Design review of the part built by this model. Coordinates are the model's own, in mm. Face numbers are marked on the shaded views. A direction names the side the tool comes from. Coordinates: 2 decimals unless noted, no trailing zeros. Write each loop counter-clockwise with the first axis right and the second up, starting at its lowest first coordinate (ties: lowest second). Pieces come first, ordered by that corner, then holes. Notation, with made-up numbers: M 74.25,16 L 118.25,16 A20 cw 118.25,37 Z; hole C 71,-16 d4. An arc over 180 degrees is marked long. Write item = value, one per line.
```python
from build123d import *

# Parameters (mm, degrees)
SKETCH1_R           = 1.8749999999999902
SKETCH1_R_2         = 1.8749999999999822
BOSS_EXTRUDE1_DEPTH = 50


with BuildPart() as part:
    # Sketch1 → Boss-Extrude1 (new body)
    # profile 1 of 3: a face of its own
    with BuildSketch(Plane.XY):
        with BuildLine():
            ThreePointArc((-544.9073445733862, 245.05934298496234), (-541.6610147269474, 238.65452406819674), (-534.9592100975257, 236.0765059267749))
            Line((-534.9592100975257, 236.07650592677487), (-441.5899759130262, 236.07650592677487))
            Line((-441.5899759130262, 236.07650592677484), (-439.06259783112466, 236.07650592677484))
            ThreePointArc((-439.06259783112466, 236.07650592677484), (-397.37358262088145, 226.97219345264216), (-363.27556383489673, 201.31702614277702))
            add(Edge.make_bspline(
                [(-383.12296849125244, 224.93458304595043), (-367.62274464990907, 206.36695430282649), (-363.27556383489645, 201.31702614277665)],
                knots=[-0.5220285895473142, -0.5220285895473142, -0.5220285895473142, 1.887e-14, 1.887e-14, 1.887e-14], degree=2))
            ThreePointArc((-383.1229684912514, 224.93458304595174), (-405.8980891559586, 235.70137914794805), (-430.5822522506289, 240.7334872459175))
            ThreePointArc((-430.5822522506289, 240.7334872459175), (-433.50085290752264, 241.98064646711703), (-435.0806969123075, 244.73341395420863))
            ThreePointArc((-435.08069691230753, 244.73341395420863), (-440.8631120126931, 249.55208851055136), (-446.8033920996223, 244.92942462898426))
            ThreePointArc((-446.8033920996222, 244.92942462898426), (-448.5664399466794, 242.15633970013647), (-451.6700341140156, 241.07650592677487))
            Line((-451.6700341140156, 241.07650592677487), (-523.9636485779045, 241.07650592677487))
            ThreePointArc((-523.9636485779045, 241.07650592677481), (-527.448607657875, 242.49111052167248), (-528.9616310868231, 245.93448184240285))
            ThreePointArc((-528.9616310868231, 245.93448184240285), (-533.6831252946306, 251.62678332689148), (-540.3433752762132, 248.41183792649997))
            ThreePointArc((-540.3433752762132, 248.41183792649997), (-541.6780229849218, 246.8731065868591), (-543.5973644050546, 246.19111893673872))
            Line((-543.5973644050546, 246.19111893673875), (-543.9963947067045, 246.15753652414114))
            ThreePointArc((-543.9963947067045, 246.15753652414116), (-544.6822020264595, 245.79950011796763), (-544.9073445733864, 245.05934298496234))
        make_face()
        with Locations((-534.9592100975258, 246.07650592677487)):
            Circle(SKETCH1_R, mode=Mode.SUBTRACT)
        with Locations((-440.9634216823502, 243.55292707163554)):
            Circle(SKETCH1_R, mode=Mode.SUBTRACT)
    # profile 2 of 3: a face of its own
    with BuildSketch(Plane.XY):
        with BuildLine():
            add(Edge.make_bspline(
                [(-383.12296849125244, 224.93458304595043), (-367.62274464990907, 206.36695430282649), (-363.27556383489645, 201.31702614277665)],
                knots=[-0.5220285895473142, -0.5220285895473142, -0.5220285895473142, 1.887e-14, 1.887e-14, 1.887e-14], degree=2))
            add(Edge.make_bspline(
                [(-363.2755638348965, 201.3170261427767), (-362.2346292716234, 200.10781838548988), (-361.83317155831753, 199.67366875065946), (-361.04162411691453, 198.81766319578747), (-360.27634316412167, 198.13844219041232), (-358.52376862577097, 196.58295405812672), (-356.6619331821235, 195.7294886371459), (-354.80036900749667, 194.8761475658919), (-352.4846532551344, 194.56947395223122), (-351.48825008923626, 194.4375188281029), (-350.30526494816087, 194.39325502601127), (-349.5536063403822, 194.3651301859774), (-348.11815703565105, 194.36513018597736)],
                knots=[1.893e-14, 1.893e-14, 1.893e-14, 0.125, 0.125, 0.25, 0.25, 0.5, 0.5, 0.75, 0.75, 0.875, 0.875, 1.0000000000000016, 1.0000000000000016, 1.0000000000000016], degree=2))
            add(Edge.make_bspline(
                [(-348.11815703565105, 194.36513018597736), (-333.4550041742609, 194.36513018597725), (-247.44050149953085, 197.29986636862012)],
                knots=[1.0000000000000016, 1.0000000000000016, 1.0000000000000016, 2.276878327665547, 2.276878327665547, 2.276878327665547], degree=2))
            ThreePointArc((-247.44050149953077, 197.29986636861926), (-230.0871000090499, 203.33834671649424), (-214.13144535031904, 212.4499257570787))
            Line((-214.13144535031904, 212.44992575707866), (-155.67654819642465, 253.3804853895092))
            ThreePointArc((-155.67654819642465, 253.3804853895092), (-154.62961317001395, 254.68034309191702), (-154.43933268041653, 256.3385036183176))
            ThreePointArc((-154.4393326804165, 256.3385036183176), (-161.0507101720321, 261.2969344989494), (-166.3426632069391, 254.94936943737002))
            ThreePointArc((-166.34266320693914, 254.94936943737002), (-166.8247741855496, 252.4619720660458), (-168.46431508885058, 250.5302675583712))
            Line((-168.46431508885058, 250.5302675583712), (-216.9993275320743, 216.5456859785236))
            ThreePointArc((-216.9993275320743, 216.5456859785236), (-237.69631255795534, 205.57859820435817), (-260.44760709280405, 200.00896622402453))
            ThreePointArc((-260.44760709280405, 200.0089662240245), (-263.72642255227106, 200.76527055587718), (-265.7834428399557, 203.42821903372513))
            ThreePointArc((-265.7834428399557, 203.42821903372513), (-271.6624634978908, 207.56948031752756), (-277.29243682695915, 203.0955190714807))
            ThreePointArc((-277.29243682695915, 203.0955190714807), (-279.07471454855846, 200.40608638901813), (-282.12856002823787, 199.36513018597742))
            Line((-282.12856002823787, 199.3651301859774), (-345.74927319295944, 199.3651301859774))
            ThreePointArc((-345.74927319295944, 199.36513018597742), (-348.8572930869804, 200.4484718732866), (-350.61849397452966, 203.22904525062938))
            ThreePointArc((-350.61849397452966, 203.22904525062938), (-353.49762862356397, 207.08255435055457), (-358.2818252430184, 207.58296559830646))
            ThreePointArc((-358.2818252430184, 207.5829655983065), (-361.0270213713086, 207.50053911285607), (-363.40161766909495, 208.88046241899406))
            ThreePointArc((-363.40161766909495, 208.88046241899406), (-372.7744857551701, 217.50675950249254), (-383.1229684912514, 224.93458304595174))
        make_face()
        with Locations((-356.46155891241386, 201.86574332821175)):
            Circle(SKETCH1_R, mode=Mode.SUBTRACT)
        with Locations((-271.4890889854247, 201.57198573408468)):
            Circle(SKETCH1_R, mode=Mode.SUBTRACT)
        with Locations((-160.35522233053905, 255.3373794264347)):
            Circle(SKETCH1_R_2, mode=Mode.SUBTRACT)
    # profile 3 of 3: a face of its own
    with BuildSketch(Plane.XY):
        with BuildLine():
            add(Edge.make_bspline(
                [(-348.11815703565105, 194.36513018597736), (-333.4550041742609, 194.36513018597725), (-247.44050149953085, 197.29986636862012)],
                knots=[1.0000000000000016, 1.0000000000000016, 1.0000000000000016, 2.276878327665547, 2.276878327665547, 2.276878327665547], degree=2))
            Line((-348.11815703565105, 194.3651301859774), (-271.4890889854247, 194.36513018597734))
            ThreePointArc((-271.4890889854247, 194.36513018597736), (-259.3755920034587, 195.10152562283494), (-247.44050149953077, 197.29986636861926))
        make_face()
    extrude(amount=BOSS_EXTRUDE1_DEPTH)


solid = part.part
```
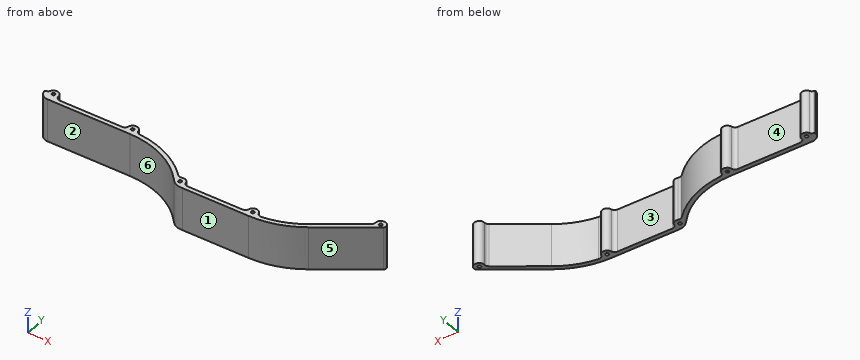
Q1. Consider section B-B, the plane z = 15. State how many separate pieces and enclosed holes the cut face has, and give its area (3 significant figures).
Check result:
separate_pieces = 1
enclosed_holes = 5
area = 2,460 mm²
Q2. Consider section C-C, the plane x = -470. State the section outline as (y, z) points.
Check result:
outline = M 236.08,0 L 241.08,0 L 241.08,50 L 236.08,50 Z
Q3. Consider section A-A, the plane y = 222.5. State the section outline as (x, z) points.
Check result:
outline = M -388.75,0 L -379.43,0 L -379.43,50 L -388.75,50 Z; M -208.5,0 L -199.78,0 L -199.78,50 L -208.5,50 Z
Q4. Machinability: for the marked faces 1, 2 and 3, which of the approach directions +Z, -Z, +X, -X, +Y, -Y give a long, thin tool a straight path to every point of the face, cutting with its end or side? Answer none if there is none.
Check result:
face_1 = +Z, -Z, +X, -X, -Y
face_2 = +Z, -Z, -X, -Y
face_3 = +Z, -Z, +Y
Q5. Consider section D-D, the plane x = -372.5. State the section outline as (y, z) points.
Check result:
outline = M 210.71,0 L 217.28,0 L 217.28,50 L 210.71,50 Z
Q6. For P1, Ø1, axis at x = -497.5, z = 26, coming from the +Y side; P2, Ø1, axis at y = 253, z = 23.5, coming from the +X side; P3, Ø6, axis at y = 215, z = 22, coming from the -X side; P4, Ø3, axis at x = -160.36, y = 255.34, coming from the -Z side, all flat-tipped, find the tip position at first contact; note any pin that passes through.
Check result:
P1 = 241.08
P2 = -155.52
P3 = -381.72
P4 = through
Q7. Wall thickness on line 1 (X direction, y = 247, z = 24.5); line 2 (X direction, y = 206.5, z = 3.5); line 3 (Y direction, x = -521, z = 25.5): over which ranges is each line inside the solid? List them lowest first.
Check result:
line_1 = -541.5 to -536.59, -533.33 to -529.09, -445.87 to -436.05, -173.51 to -164.79
line_2 = -368.07 to -352.65, -274.91 to -268.07, -235.37 to -223.74
line_3 = 236.08 to 241.08
Q8. The part is to be moulded in two halves that separate along X. For the marked faces 4, 5 and 6, say which applies: +X half, -X half, draft (parallel to the pull), parting line (faces both ways), or undercut.
Check result:
face_4 = undercut
face_5 = +X half
face_6 = -X half
